from build123d import *

# Parameters (mm, degrees)
EXTRUDE_1_DEPTH     = 20.2
SKETCH_4_W          = 4.5
SKETCH_4_H          = 1.2
CUT_EXTRUDE_1_DEPTH = 10
SKETCH_5_W          = 4.5
SKETCH_5_H          = 10
CUT_EXTRUDE_2_DEPTH = 10
SKETCH_6_W          = 5
SKETCH_6_H          = 5
EXTRUDE_2_DEPTH     = 1.4
SKETCH_7_W          = 7.6
SKETCH_7_H          = 2.5
CUT_EXTRUDE_3_DEPTH = 5
SKETCH_8_R          = 1
CUT_EXTRUDE_4_DEPTH = 5
SKETCH_9_R          = 2
CUT_EXTRUDE_5_DEPTH = 1.5
CUT_EXTRUDE_6_DEPTH = 5
CUT_EXTRUDE_7_DEPTH = 5
SKETCH_12_R         = 1
SKETCH_12_R_2       = 0.925
EXTRUDE_3_DEPTH     = 1.5
SKETCH_13_W         = 10
SKETCH_13_H         = 2.102852528
CUT_EXTRUDE_8_DEPTH = 0.2
SKETCH_14_W         = 10
SKETCH_14_H         = 2.102852528
CUT_EXTRUDE_9_DEPTH = 0.2
FILLET_2_R          = 1
EXTRUDE_START       = 0.5
SKETCH_15_R         = 0.925
EXTRUDE_4_DEPTH     = 0.5
SKETCH_16_W         = 5
SKETCH_16_H         = 10.2
EXTRUDE_5_DEPTH     = 0.2


with BuildPart() as part:
    # 草图3 → 凸台-拉伸1 (new body)
    with BuildSketch(Plane.XY):
        with BuildLine():
            Line((-10.1, 22), (10.1, 22))
            ThreePointArc((10.1, 22), (0, 24.207643421), (-10.1, 22))
        make_face()
    extrude(amount=EXTRUDE_1_DEPTH)

    # 草图4 → 切除-拉伸1 (cut)
    with BuildSketch(Plane(origin=(6.414908285, -11.03, 20.2), x_dir=(1, 0, 0), z_dir=(0, 0, 1))):
        with Locations((-6.414908285, 33.63)):
            Rectangle(SKETCH_4_W, SKETCH_4_H)
    extrude(amount=-CUT_EXTRUDE_1_DEPTH, mode=Mode.SUBTRACT)

    # 草图5 → 切除-拉伸2 (cut)
    with BuildSketch(Plane.XZ.offset(-23.2)):
        with Locations((0, 15.2)):
            Rectangle(SKETCH_5_W, SKETCH_5_H)
    extrude(amount=-CUT_EXTRUDE_2_DEPTH, mode=Mode.SUBTRACT)

    # 草图6 → 凸台-拉伸2 (add)
    with BuildSketch(Plane.XZ.offset(-22)):
        with Locations((-7.6, 17.7)):
            Rectangle(SKETCH_6_W, SKETCH_6_H)
        with Locations((-7.6, 2.5)):
            Rectangle(SKETCH_6_W, SKETCH_6_H)
        with Locations((7.6, 2.5)):
            Rectangle(SKETCH_6_W, SKETCH_6_H)
        with Locations((7.6, 17.7)):
            Rectangle(SKETCH_6_W, SKETCH_6_H)
    extrude(amount=EXTRUDE_2_DEPTH)

    # 草图7 → 切除-拉伸3 (cut)
    with BuildSketch(Plane(origin=(6.414908285, -11.03, 0), x_dir=(1, 0, 0), z_dir=(0, 0, -1))):
        with Locations((-6.414908285, -32.88)):
            Rectangle(SKETCH_7_W, SKETCH_7_H)
    extrude(amount=-CUT_EXTRUDE_3_DEPTH, mode=Mode.SUBTRACT)

    # 草图8 → 切除-拉伸4 (cut)
    with BuildSketch(Plane(origin=(6.414908285, 20.6, 10.797250082), x_dir=(-1, 0, 0), z_dir=(0, -1, 0))):
        with Locations(Location((13.914908285, -6.802749918, 0), (0, 0, 90))):
            Circle(SKETCH_8_R)
        with Locations(Location((-1.085091715, -6.802749918, 0), (0, 0, 90))):
            Circle(SKETCH_8_R)
        with Locations(Location((-1.085091715, 8.197250082, 0), (0, 0, 90))):
            Circle(SKETCH_8_R)
        with Locations(Location((13.914908285, 8.197250082, 0), (0, 0, 90))):
            Circle(SKETCH_8_R)
    extrude(amount=-CUT_EXTRUDE_4_DEPTH, mode=Mode.SUBTRACT)

    # 草图9 → 切除-拉伸5 (cut)
    with BuildSketch(Plane(origin=(0, 23.6, 0), x_dir=(-1, 0, 0), z_dir=(0, -1, 0))):
        with Locations(Location((7.5, -2.6, 0), (0, 0, 270))):
            Circle(SKETCH_9_R)
        with Locations(Location((-7.5, -2.6, 0), (0, 0, 270))):
            Circle(SKETCH_9_R)
        with Locations(Location((7.5, -17.6, 0), (0, 0, 270))):
            Circle(SKETCH_9_R)
        with Locations(Location((-7.5, -17.6, 0), (0, 0, 270))):
            Circle(SKETCH_9_R)
    extrude(amount=CUT_EXTRUDE_5_DEPTH, mode=Mode.SUBTRACT)

    # 草图10 → 切除-拉伸6 (cut)
    with BuildSketch(Plane(origin=(6.414908285, 22, 10.797250082), x_dir=(-1, 0, 0), z_dir=(0, -1, 0))):
        with BuildLine():
            Line((7.57208535, 2.759943394), (3.695561186, 6.636467557))
            ThreePointArc((3.695561186, 6.636467557), (3.641367999, 6.908915111), (3.872337882, 7.063244252))
            Line((3.872337882, 7.063244252), (4.354570929, 7.063244252))
            ThreePointArc((4.354570929, 7.063244252), (4.737254361, 6.987123785), (5.06167771, 6.770351034))
            Line((5.06167771, 6.770351034), (8.938201874, 2.89382687))
            ThreePointArc((8.938201874, 2.89382687), (8.992395061, 2.621379317), (8.761425178, 2.467050175))
            Line((8.761425178, 2.467050175), (8.279192131, 2.467050175))
            ThreePointArc((8.279192131, 2.467050175), (7.896508699, 2.543170642), (7.57208535, 2.759943394))
        make_face()
        with BuildLine():
            Line((4.965840766, 4.305527806), (6.003708732, 3.26765984))
            ThreePointArc((6.003708732, 3.26765984), (6.047642714, 3.161593823), (6.003708732, 3.055527806))
            Line((6.003708732, 3.055527806), (5.182998054, 2.234817128))
            ThreePointArc((5.182998054, 2.234817128), (4.858574705, 2.018044376), (4.475891272, 1.941923909))
            Line((4.475891272, 1.941923909), (2.993658225, 1.941923909))
            ThreePointArc((2.993658225, 1.941923909), (2.762688342, 2.096253051), (2.81688153, 2.368700604))
            Line((2.81688153, 2.368700604), (4.753708732, 4.305527806))
            ThreePointArc((4.753708732, 4.305527806), (4.859774749, 4.349461789), (4.965840766, 4.305527806))
        make_face()
        with BuildLine():
            Line((7.814368903, 5.078320012), (6.776500938, 6.116187978))
            ThreePointArc((6.776500938, 6.116187978), (6.732566955, 6.222253995), (6.776500938, 6.328320012))
            Line((6.776500938, 6.328320012), (8.097211616, 7.64903069))
            ThreePointArc((8.097211616, 7.64903069), (8.421634965, 7.865803441), (8.804318397, 7.941923909))
            Line((8.804318397, 7.941923909), (10.286551444, 7.941923909))
            ThreePointArc((10.286551444, 7.941923909), (10.517521327, 7.787594767), (10.463328139, 7.515147214))
            Line((10.463328139, 7.515147214), (8.026500938, 5.078320012))
            ThreePointArc((8.026500938, 5.078320012), (7.920434921, 5.034386029), (7.814368903, 5.078320012))
        make_face()
    extrude(amount=-CUT_EXTRUDE_6_DEPTH, mode=Mode.SUBTRACT)

    # 草图11 → 切除-拉伸7 (cut)
    with BuildSketch(Plane(origin=(6.414908285, 20.6, 10.797250082), x_dir=(-1, 0, 0), z_dir=(0, -1, 0))):
        with BuildLine():
            Line((16.514908285, -9.402749918), (16.514908285, -8.402749918))
            ThreePointArc((16.514908285, -8.402749918), (16.222015066, -9.109856699), (15.514908285, -9.402749918))
            Line((15.514908285, -9.402749918), (16.514908285, -9.402749918))
        make_face()
        with BuildLine():
            Line((-3.685091715, -9.402749918), (-2.685091715, -9.402749918))
            ThreePointArc((-2.685091715, -9.402749918), (-3.392198496, -9.109856699), (-3.685091715, -8.402749918))
            Line((-3.685091715, -8.402749918), (-3.685091715, -9.402749918))
        make_face()
        with BuildLine():
            Line((-3.685091715, 10.797250082), (-3.685091715, 9.797250082))
            ThreePointArc((-3.685091715, 9.797250082), (-3.392198496, 10.504356863), (-2.685091715, 10.797250082))
            Line((-2.685091715, 10.797250082), (-3.685091715, 10.797250082))
        make_face()
        with BuildLine():
            Line((16.514908285, 10.797250082), (15.514908285, 10.797250082))
            ThreePointArc((15.514908285, 10.797250082), (16.222015066, 10.504356863), (16.514908285, 9.797250082))
            Line((16.514908285, 9.797250082), (16.514908285, 10.797250082))
        make_face()
    extrude(amount=-CUT_EXTRUDE_7_DEPTH, mode=Mode.SUBTRACT)

    # 草图12 → 凸台-拉伸3 (add)
    # profile 1 of 4: a face of its own
    with BuildSketch(Plane.XZ.offset(-20.6)):
        with Locations((7.5, 17.6)):
            Circle(SKETCH_12_R)
        with Locations(Location((7.5, 17.6, 0), (0, 0, 270))):
            Circle(SKETCH_12_R_2, mode=Mode.SUBTRACT)
    # profile 2 of 4: a face of its own
    with BuildSketch(Plane.XZ.offset(-20.6)):
        with Locations((-7.5, 17.6)):
            Circle(SKETCH_12_R)
        with Locations(Location((-7.5, 17.6, 0), (0, 0, 270))):
            Circle(SKETCH_12_R_2, mode=Mode.SUBTRACT)
    # profile 3 of 4: a face of its own
    with BuildSketch(Plane.XZ.offset(-20.6)):
        with Locations((-7.5, 2.6)):
            Circle(SKETCH_12_R)
        with Locations(Location((-7.5, 2.6, 0), (0, 0, 270))):
            Circle(SKETCH_12_R_2, mode=Mode.SUBTRACT)
    # profile 4 of 4: a face of its own
    with BuildSketch(Plane.XZ.offset(-20.6)):
        with Locations((7.5, 2.6)):
            Circle(SKETCH_12_R)
        with Locations(Location((7.5, 2.6, 0), (0, 0, 270))):
            Circle(SKETCH_12_R_2, mode=Mode.SUBTRACT)
    extrude(amount=-EXTRUDE_3_DEPTH)

    # 草图13 → 切除-拉伸8 (cut)
    with BuildSketch(Plane.ZY.offset(-2.25)):
        with Locations((15.2, 23.051426264)):
            Rectangle(SKETCH_13_W, SKETCH_13_H)
    extrude(amount=-CUT_EXTRUDE_8_DEPTH, mode=Mode.SUBTRACT)

    # 草图14 → 切除-拉伸9 (cut)
    with BuildSketch(Plane(origin=(-2.25, 0, 0), x_dir=(0, 0, -1), z_dir=(1, 0, 0))):
        with Locations((-15.2, 23.051426264)):
            Rectangle(SKETCH_14_W, SKETCH_14_H)
    extrude(amount=-CUT_EXTRUDE_9_DEPTH, mode=Mode.SUBTRACT)

    # 圆角2
    fillet_2_edges = [part.edges().sort_by_distance(p)[0] for p in [
        (2.45, 23.041672434, 10.2),
        (-2.45, 23.041672434, 10.2),
    ]]
    fillet(fillet_2_edges, radius=FILLET_2_R)

    # 草图15 → 凸台-拉伸4 (add)
    # profile 1 of 4: a face of its own
    with BuildSketch(Plane.XZ.offset(-20.6).offset(EXTRUDE_START)):
        with BuildLine():
            Line((-10.1, 5), (-10.1, 1))
            ThreePointArc((-10.1, 1), (-9.807106781, 0.292893219), (-9.1, 0))
            Line((-9.1, 0), (-5.1, 0))
            Line((-5.1, 0), (-5.1, 5))
            Line((-5.1, 5), (-10.1, 5))
        make_face()
        with Locations(Location((-7.5, 2.6, 0), (0, 0, 270))):
            Circle(SKETCH_15_R, mode=Mode.SUBTRACT)
    # profile 2 of 4: a face of its own
    with BuildSketch(Plane.XZ.offset(-20.6).offset(EXTRUDE_START)):
        with BuildLine():
            Line((-10.1, 19.2), (-10.1, 15.2))
            Line((-10.1, 15.2), (-5.1, 15.2))
            Line((-5.1, 15.2), (-5.1, 20.2))
            Line((-5.1, 20.2), (-9.1, 20.2))
            ThreePointArc((-9.1, 20.2), (-9.807106781, 19.907106781), (-10.1, 19.2))
        make_face()
        with Locations(Location((-7.5, 17.6, 0), (0, 0, 270))):
            Circle(SKETCH_15_R, mode=Mode.SUBTRACT)
    # profile 3 of 4: a face of its own
    with BuildSketch(Plane.XZ.offset(-20.6).offset(EXTRUDE_START)):
        with BuildLine():
            Line((9.1, 20.2), (5.1, 20.2))
            Line((5.1, 20.2), (5.1, 15.2))
            Line((5.1, 15.2), (10.1, 15.2))
            Line((10.1, 15.2), (10.1, 19.2))
            ThreePointArc((10.1, 19.2), (9.807106781, 19.907106781), (9.1, 20.2))
        make_face()
        with Locations(Location((7.5, 17.6, 0), (0, 0, 270))):
            Circle(SKETCH_15_R, mode=Mode.SUBTRACT)
    # profile 4 of 4: a face of its own
    with BuildSketch(Plane.XZ.offset(-20.6).offset(EXTRUDE_START)):
        with BuildLine():
            Line((5.1, 0), (9.1, 0))
            ThreePointArc((9.1, 0), (9.807106781, 0.292893219), (10.1, 1))
            Line((10.1, 1), (10.1, 5))
            Line((10.1, 5), (5.1, 5))
            Line((5.1, 5), (5.1, 0))
        make_face()
        with Locations(Location((7.5, 2.6, 0), (0, 0, 270))):
            Circle(SKETCH_15_R, mode=Mode.SUBTRACT)
    extrude(amount=-EXTRUDE_4_DEPTH)

    # 草图16 → 凸台-拉伸5 (add)
    with BuildSketch(Plane.XZ.offset(-22)):
        with Locations((-7.6, 10.1)):
            Rectangle(SKETCH_16_W, SKETCH_16_H)
        with Locations((7.6, 10.1)):
            Rectangle(SKETCH_16_W, SKETCH_16_H)
    extrude(amount=EXTRUDE_5_DEPTH)


solid = part.part
Verification items for the finished model (mm, model axes). A direction names the side the tool comes from. Round coordinates to 2 decimals unless told otherwise and drop trailing zeros. Loops run counter-clockwise (first coordinate to the right, second up) from the corner with the lowest first, then second, coordinate; pieces in that order, holes last. Notation, with made-up numbers: (-30.75, 53.5) - (-21.75, 53.5) arc R4 ccw to (-21.75, 58.5) - close; hole circle Ø11 at (86, -39). An arc over 180 degrees is marked (long way). Answer in a Markdown table with one row per item. Add a question column.
Q1. Material ranges on line 1 (X direction, y = 21.6, z = 2.6) (3 decimals); line 2 (Z direction, x = -7.5, y = 22.3); line 3 (X direction, y = 22.5, z = 17.6), recorded low to high.
Q2. Tool access check on faces 1 (the face through (9.815, 21.25, 0.301)), 2 (the face through (-3.8, 22.6, 4.3)), 3 (the face through (2.45, 23, 16)), 4 (the face through (5.517, 22.684, 17.34)), 5 (the face through (0.94, 23.09, 7)). Record the directions out of +Z, -Z, +X, -X, +Y, -Y that give a thin tool (end or side, any length) a straight path to the whole face; none if there is none.
Q3. Section check C-C on x = 7.5. Enter the section's corners in (y, z) (3 decimals), plus the area to 3 significant figures.
Q4. Section check A-A on y = 20.85. Enter the section's corners in (x, z) (3 decimals), plus the area to 3 significant figures.
Q5. Section check B-B on z = 17.5. Enter the section's corners in (x, y), plus the area to 3 significant figures.
Q6. Section check D-D on z = 2.6. Enter the section's corners in (x, y) (3 decimals), plus the area to 3 significant figures.
Q7. Gauge pin test, flat ends, axial feed: pin 1 (3 mm diameter, centred on x = 2, z = 9.5, fed in from -Y); pin 2 (1.2 mm diameter, centred on x = -7, z = 2, fed in from +Y); pin 3 (1.5 mm diameter, centred on y = 23, z = 4, fed in from -X); pin 4 (1 mm diameter, centred on x = -3.5, y = 20.5, fed in from +Z). Record the tip position at first contact, or that the pin passes through.
Q8. Release check for a two-part mould opening along X. For faces 6 (the face through (-10.1, 21, 16)), 7 (the face through (0, 23.1, 2)), 8 (the face through (-9, 20.1, 18)), 9 (the face through (10.1, 21, 16)) record: pulls with the +X half, pulls with the -X half, needs draft (parallel to the pull), parting line crosses it, or undercut.
Found:
| question | item | result |
|---|---|---|
| 1 | line 1 | x = -10.1 to -8.425, -6.575 to -5.1, 5.1 to 6.575, 8.425 to 10.1 |
| 1 | line 2 | z = 0 to 0.6, 4.6 to 15.6, 19.6 to 20.2 |
| 1 | line 3 | x = -5.5 to -2.45, 2.45 to 5.5 |
| 2 | face 1 | -Z, +X, +Y, -Y |
| 2 | face 2 | -Z, -Y |
| 2 | face 3 | +Z, +Y, -Y |
| 2 | face 4 | +Y |
| 2 | face 5 | +Y, -Y |
| 3 | outline | (20.1, 0) - (23.017, 0) - (23.017, 0.6) - (22.1, 0.6) - (22.1, 1.675) - (20.1, 1.675) - close; (20.1, 3.525) - (22.1, 3.525) - (22.1, 4.6) - (23.017, 4.6) - (23.017, 15.6) - (22.1, 15.6) - (22.1, 16.675) - (20.1, 16.675) - (20.1, 15.2) - (21.8, 15.2) - (21.8, 5) - (20.1, 5) - close; (20.1, 18.525) - (22.1, 18.525) - (22.1, 19.6) - (23.017, 19.6) - (23.017, 20.2) - (20.1, 20.2) - close |
| 3 | area | 26.8 mm² |
| 4 | outline | (-10.1, 1) arc R1 ccw to (-9.1, 0) - (-5.1, 0) - (-5.1, 5) - (-10.1, 5) - close; (-10.1, 15.2) - (-5.1, 15.2) - (-5.1, 20.2) - (-9.1, 20.2) arc R1 ccw to (-10.1, 19.2) - close; (5.1, 0) - (9.1, 0) arc R1 ccw to (10.1, 1) - (10.1, 5) - (5.1, 5) - close; (5.1, 15.2) - (10.1, 15.2) - (10.1, 19.2) arc R1 ccw to (9.1, 20.2) - (5.1, 20.2) - close; hole circle Ø1.85 at (-7.5, 2.6); hole circle Ø1.85 at (-7.5, 17.6); hole circle Ø1.85 at (7.5, 2.6); hole circle Ø1.85 at (7.5, 17.6) |
| 4 | area | 88.4 mm² |
| 5 | outline | (-10.1, 20.1) - (-8.42, 20.1) - (-8.42, 22.1) - (-9.5, 22.1) - (-9.5, 22.27) arc R24.21 ccw to (-10.1, 22) - close; (-6.58, 20.1) - (-5.1, 20.1) - (-5.1, 22) - (-2.45, 22) - (-2.45, 24.08) arc R24.21 ccw to (-5.5, 23.57) - (-5.5, 22.1) - (-6.58, 22.1) - close; (2.45, 22) - (5.1, 22) - (5.1, 20.1) - (6.58, 20.1) - (6.58, 22.1) - (5.5, 22.1) - (5.5, 23.57) arc R24.21 ccw to (2.45, 24.08) - close; (8.42, 20.1) - (10.1, 20.1) - (10.1, 22) arc R24.21 ccw to (9.5, 22.27) - (9.5, 22.1) - (8.42, 22.1) - close |
| 5 | area | 24.0 mm² |
| 6 | outline | (-10.1, 20.1) - (-8.425, 20.1) - (-8.425, 22.1) - (-9.5, 22.1) - (-9.5, 22.266) arc R24.208 ccw to (-10.1, 22) - close; (-6.575, 20.1) - (-5.1, 20.1) - (-5.1, 22) - (-3.8, 22) - (-3.8, 23.1) - (3.8, 23.1) - (3.8, 22) - (5.1, 22) - (5.1, 20.1) - (6.575, 20.1) - (6.575, 22.1) - (5.5, 22.1) - (5.5, 23.575) arc R24.208 ccw to (-5.5, 23.575) - (-5.5, 22.1) - (-6.575, 22.1) - close; (8.425, 20.1) - (10.1, 20.1) - (10.1, 22) arc R24.208 ccw to (9.5, 22.266) - (9.5, 22.1) - (8.425, 22.1) - close |
| 6 | area | 26.2 mm² |
| 7 | pin 1 | stops at y = 22 |
| 7 | pin 2 | stops at y = 22.1 |
| 7 | pin 3 | stops at x = -9.54 |
| 7 | pin 4 | passes through |
| 8 | face 6 | pulls with the -X half |
| 8 | face 7 | undercut |
| 8 | face 8 | needs draft |
| 8 | face 9 | pulls with the +X half |
